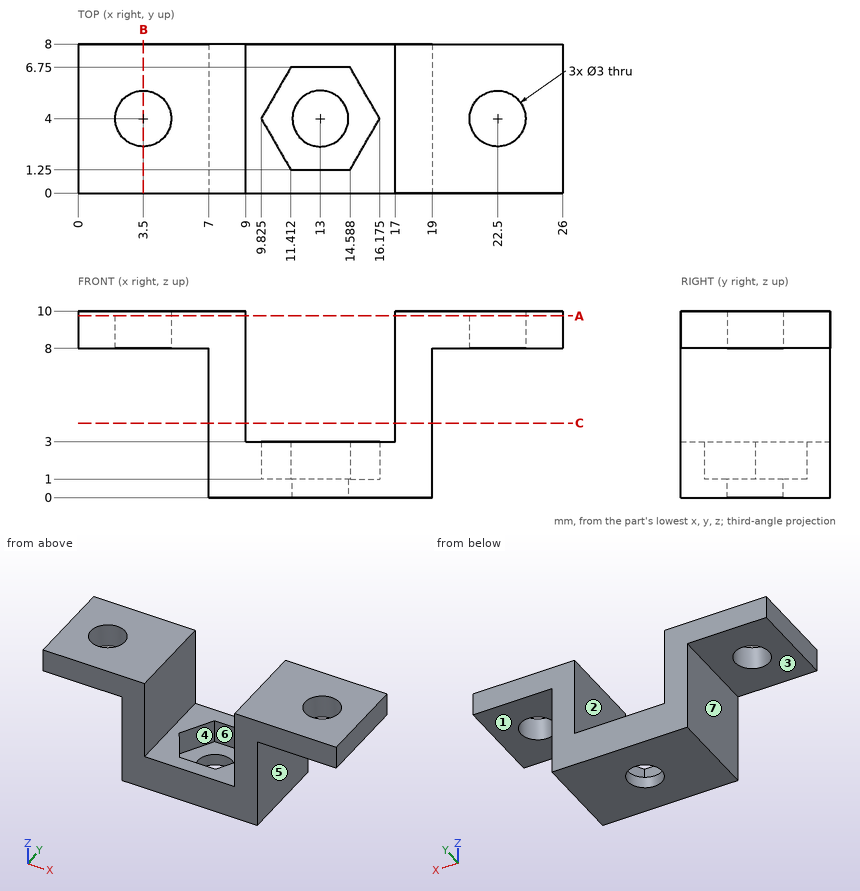
Print and shaded views of the part. All mm, measured from the part's lowest x, y and z. A direction names the side the tool comes from. Coordinates: 2 decimals unless noted, no trailing zeros. Order: outer loops, then holes, each group sorted by start corner. A loop starts at its lowest first (then second) coordinate and runs counter-clockwise, first axis right, second up. Notation, with made-up numbers: (-1, 33) - (43, 33) arc R15 cw to (43, 52) - close; hole circle Ø9 at (-13.75, 17). An arc over 180 degrees is marked (long way). Put each result on its own line as item: value.
1. Saw through at C-C (z = 4). Write the cut outline in (x, y), and give its area (3 significant figures).
Answer sheet:
outline: (7, 0) - (9, 0) - (9, 8) - (7, 8) - close; (17, 0) - (19, 0) - (19, 8) - (17, 8) - close
area: 32.0 mm^2
2. Saw through at B-B (x = 3.5). Write the cut outline in (y, z).
Answer sheet:
outline: (0, 8) - (2.5, 8) - (2.5, 10) - (0, 10) - close; (5.5, 8) - (8, 8) - (8, 10) - (5.5, 10) - close
3. Probe line 1 along X through (y, z) = (6.5, 6.75); line 2 along Y through (x, z) = (22.5, 8.4); line 3 along Z through (x, y) = (3.5, 6.5). List the from-to ranges inside material, lowest first. Write a range as [from, to].
Answer sheet:
line 1: x = [7, 9], [17, 19]
line 2: y = [0, 2.5], [5.5, 8]
line 3: z = [8, 10]
4. Tool access for the marked faces 1, 2, 3 and 4: list every direction of +Z, -Z, +X, -X, +Y, -Y with a clear straight run to the whole face (end or side of a thin tool).
Answer sheet:
face 1: -Z, +X, +Y, -Y
face 2: +Z, +Y, -Y
face 3: -Z, -X, +Y, -Y
face 4: +Z
5. Drop flat-ended pins along their axis: P1, Ø3, axis at y = 1, z = 3, coming from the -X side; P2, Ø1.6, axis at x = 12, y = 4, coming from the +Z side; P3, Ø2, axis at y = 5.5, z = 6.5, coming from the +X side. Give the stop position or say it passes through.
Answer sheet:
P1: stops at x = 7
P2: stops at z = 1
P3: stops at x = 19
6. Pull direction X, two halves, no side cores. Call the marked faces 5, 6 and 7: pulls with the +X half, pulls with the -X half, needs draft (parallel to the pull), parting line crosses it, or undercut.
Answer sheet:
face 5: pulls with the +X half
face 6: undercut
face 7: pulls with the -X half
7. Saw through at A-A (z = 9.75). Write the cut outline in (x, y), and give its area (3 significant figures).
Answer sheet:
outline: (0, 0) - (9, 0) - (9, 8) - (0, 8) - close; (17, 0) - (26, 0) - (26, 8) - (17, 8) - close; hole circle Ø3 at (3.5, 4); hole circle Ø3 at (22.5, 4)
area: 130 mm^2
